Geometry: final body of the model. Coordinates: model frame, mm. Round coordinates to 2 decimals unless told otherwise and drop trailing zeros. Order: outer loops, then holes, each group sorted by start corner. A loop starts at its lowest first (then second) coordinate and runs counter-clockwise, first axis right, second up. Notation, with made-up numbers: M 55,21.5 L 103,21.5 A24 ccw 103,32.5 Z; hole C 49.25,33.5 d2. An arc over 180 degrees is marked long. Put each result on its own line as item: value. Start each with the question number.
1) Section B-B, the plane x = 7.25. Return loops of the section in (y, z) (1 decimal), then the cut area to 3 significant figures.
2) Section A-A, the plane y = -0.7. Return loops of the section in (x, z) (3 decimals).
3) Material intervals for probe 1 along Z at (x, y) = (-0.25, -3.45) (3 decimals); probe 2 along Z at (x, y) = (0.5, -1.3) (3 decimals); probe 3 along X at (y, z) = (-1.2, 18.5), sorted ascending. Write a range as [from, to].
4) Section C-C, the plane z = 15. Return loops of the section in (x, y).
from build123d import *

# Parameters (mm, degrees)
F0_W     = 25.4
F0_H     = 44.45
F1_DEPTH = 4.7625
F2_R     = 0.381
F3_R     = 19.05


with BuildPart() as f1:
    # F0 (on Front) → F1 (new body)
    with BuildSketch(Plane.XZ):
        Rectangle(F0_W, F0_H)
    extrude(amount=F1_DEPTH)

    # F2
    f2_edges = [f1.edges().sort_by_distance(p)[0] for p in [
        (-12.7, -2.38125, -22.225),
        (12.7, -2.38125, -22.225),
        (-12.7, -2.38125, 22.225),
    ]]
    fillet(f2_edges, radius=F2_R)

    # F3
    f3_edges = [f1.edges().sort_by_distance(p)[0] for p in [
        (12.7, -2.38125, 22.225),
    ]]
    fillet(f3_edges, radius=F3_R)


solid = f1.part
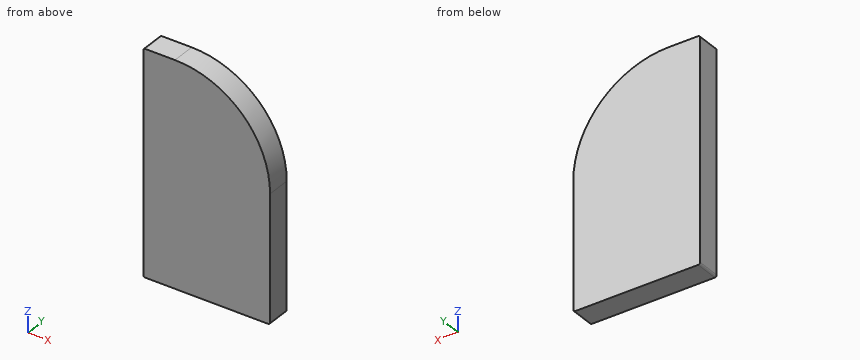
Result sheet:
1. outline: M -4.8,-22.2 L 0,-22.2 L 0,16.5 L -4.8,16.5 Z
1. area: 184 mm2
2. outline: M -12.7,-21.844 A0.381 ccw -12.319,-22.225 L 12.319,-22.225 A0.381 ccw 12.7,-21.844 L 12.7,3.175 A19.05 ccw -6.35,22.225 L -12.319,22.225 A0.381 ccw -12.7,21.844 Z
3. probe 1: z = [-22.225, 21.222]
3. probe 2: z = [-22.225, 20.951]
3. probe 3: x = [-12.7, 4.97]
4. outline: M -12.7,-4.76 L 8.59,-4.76 L 8.59,0 L -12.7,0 Z
